from build123d import *

# Parameters (mm, degrees)
F1_DEPTH    = 5
F3_DEPTH    = 5
F4_R        = 2.5
F5_DEPTH    = 25
F6_R        = 6
F7_R        = 1.5
F8_DEPTH    = 25
F9_R        = 20
F10_SIZE2   = 15
F10_SIZE    = 5
F10_2_SIZE2 = 15
F10_2_SIZE  = 5
F11_R       = 8


with BuildPart() as f1:
    # F0 (on Top) → F1 (new body)
    with BuildSketch(Plane.XY):
        Polygon((-59, 0), (0, 0), (0, 5), (-46, 5), (-46, 20), (-59, 20), align=None)
        Polygon((0, 5), (0, 0), (59, 0), (59, 20), (46, 20), (46, 5), align=None)
    extrude(amount=F1_DEPTH)

    # F2 (on Front) → F3 (join)
    with BuildSketch(Plane.XZ):
        Polygon((0, 10), (0, 0), (15, 0), (10, 10), align=None)
        Polygon((-15, 0), (0, 0), (0, 10), (-10, 10), align=None)
    extrude(amount=-F3_DEPTH)

    # F4 (on face) → F5 (cut)
    with BuildSketch(Plane(origin=(0, 5, 0), x_dir=(-1, 0, 0), z_dir=(0, 1, 0))):
        with Locations((0, 5)):
            Circle(F4_R)
    extrude(amount=-F5_DEPTH, mode=Mode.SUBTRACT)

    # F6
    f6_edges = [f1.edges().sort_by_distance(p)[0] for p in [
        (59, 20, 2.5),
        (46, 20, 2.5),
        (-46, 20, 2.5),
        (-59, 20, 2.5),
    ]]
    fillet(f6_edges, radius=F6_R)

    # F7 (on face) → F8 (cut)
    with BuildSketch(Plane.XY.offset(5)):
        with Locations((52.5, 12.5)):
            Circle(F7_R)
        with Locations((-52.5, 10.5117103085)):
            Circle(F7_R)
    extrude(amount=-F8_DEPTH, mode=Mode.SUBTRACT)

    # F9
    f9_edges = [f1.edges().sort_by_distance(p)[0] for p in [
        (46, 5, 2.5),
        (-46, 5, 2.5),
    ]]
    fillet(f9_edges, radius=F9_R)

    # F10
    f10_edges = [f1.edges().sort_by_distance(p)[0] for p in [
        (59, 0, 2.5),
    ]]
    f10_side = f1.faces().sort_by_distance((59, 7, 2.5))[0]
    chamfer(f10_edges, length=F10_SIZE, length2=F10_SIZE2, reference=f10_side)

    # F10#2
    f10_2_edges = [f1.edges().sort_by_distance(p)[0] for p in [
        (-59, 0, 2.5),
    ]]
    f10_2_side = f1.faces().sort_by_distance((-59, 7, 2.5))[0]
    chamfer(f10_2_edges, length=F10_2_SIZE, length2=F10_2_SIZE2, reference=f10_2_side)

    # F11
    f11_edges = [f1.edges().sort_by_distance(p)[0] for p in [
        (59, 5, 2.5),
        (44, 0, 2.5),
        (-44, 0, 2.5),
        (-59, 5, 2.5),
    ]]
    fillet(f11_edges, radius=F11_R)


solid = f1.part
Build history of the part. All positions in model axes, mm. A direction names the side the tool comes from. Round coordinates to 2 decimals unless told otherwise and drop trailing zeros. Loops run counter-clockwise (first coordinate to the right, second up) from the corner with the lowest first, then second, coordinate; pieces in that order, holes last. Notation, with made-up numbers: (76, 86.25) -> (133, 86.25) arc R13 cw to (133, 111.25) -> close; hole circle Ø8 at (-36, -14). An arc over 180 degrees is marked (long way). One line per item, written item: value. Start each with the question number.
Q1. Probe line 1 along Z through (x, y) = (0, 1.15); line 2 along Y through (x, z) = (-52.5, 1.5); line 3 along X through (y, z) = (18.25, 2). List the from-to ranges inside material, lowest first.
Q2. 3-axis set-ups, long thin cutter, end or side, ignore diameter. For faces 1 (the face through (48.737, 19.035, 2.535)), 2 (the face through (57.289, 18.196, 2.535)): which of +Z, -Z, +X, -X, +Y, -Y reach the whole face in a straight line?
Q3. Drop flat-ended pins along their axis: pin 1 Ø3 at (x, z) = (-27.5, 2.5) entering from +Y; pin 2 Ø6 at (x, y) = (44.5, 10.5) entering from +Z; pin 3 Ø5 at (x, y) = (-17.5, 5.5) entering from -Z. Give the stop position or say it passes through.
Q4. Cut at B-B on z = 6. List the corners of the cut face in (x, y), plus the area to 3 significant figures.
Q5. Cut at A-A on x = 0. List the corners of the cut face in (y, z), plus the area to 3 significant figures.
Q6. Two-plate mould, pull along X, no slides. Class faces 3 (the face through (41, 8, 5)), 4 (the face through (-57.449, 6.032, 2.535)), 5 (the face through (-48.82, 19.09, 2.54)): released by +X, released by -X, zero draft, split by the parting line, or undercut.
Computed:
1. line 1: 0 to 2.5, 7.5 to 10
1. line 2: 2.83 to 9.01, 12.01 to 20
1. line 3: -57.24 to -47.76, 47.76 to 57.24
2. face 1: +Z, -Z, +Y
2. face 2: +Z, -Z, +X, +Y
3. pin 1: y = 5.01
3. pin 2: z = 5
3. pin 3: z = 0
4. outline: (-12, 0) -> (-2.29, 0) -> (-2.29, 5) -> (-12, 5) -> close; (2.29, 0) -> (12, 0) -> (12, 5) -> (2.29, 5) -> close
4. area: 97.1 mm²
5. outline: (0, 0) -> (5, 0) -> (5, 2.5) -> (0, 2.5) -> close; (0, 7.5) -> (5, 7.5) -> (5, 10) -> (0, 10) -> close
5. area: 25.0 mm²
6. face 3: zero draft
6. face 4: released by -X
6. face 5: undercut
